```python
from build123d import *

# Parameters (mm, degrees)
F1_DEPTH = 5.08
F3_DEPTH = 751.84


with BuildPart() as f1:
    # F0 (on Front) → F1 (new body)
    with BuildSketch(Plane.XZ):
        Polygon((0, 482.6), (0, 0), (647.7, 0), (647.7, 504.825), align=None)
    extrude(amount=-F1_DEPTH)

    # F2 (on face) → F3 (cut)
    with BuildSketch(Plane.YZ.offset(647.7)):
        Polygon((5.08, 1.116884), (3.951849, 0), (5.08, 0), align=None)
        Polygon((0, 1.122531), (0, 0), (1.122533, 0), align=None)
    extrude(amount=-F3_DEPTH, mode=Mode.SUBTRACT)


solid = f1.part
```
Geometry: final body of the model. Coordinates: model frame, mm. Round coordinates to 2 decimals unless told otherwise and drop trailing zeros. Loops run counter-clockwise (first coordinate to the right, second up) from the corner with the lowest first, then second, coordinate; pieces in that order, holes last.
Item 1: Section B-B, the plane y = 2.95. Output: boundary loops of the cut face in (x, z) (3 decimals), plus the area to 3 significant figures.
Checked values:
outline: (0, 0) - (647.7, 0) - (647.7, 504.825) - (0, 482.6) - close
area: 320,000 mm2
Item 2: Section C-C, the plane x = 230.5. Output: boundary loops of the cut face in (y, z), plus the area to 3 significant figures.
Checked values:
outline: (0, 1.12) - (1.12, 0) - (3.95, 0) - (5.08, 1.12) - (5.08, 490.51) - (0, 490.51) - close
area: 2,490 mm2
Item 3: Line query: L1, parallel to Z at x = 268, y = 3.4; L2, parallel to Z at x = 55.5, y = 3.2. Output: solid intervals per line, ascending.
Checked values:
L1: z = 0 to 491.8
L2: z = 0 to 484.5
Item 4: Section A-A, the plane x = 304. Output: boundary loops of the cut face in (y, z).
Checked values:
outline: (0, 1.12) - (1.12, 0) - (3.95, 0) - (5.08, 1.12) - (5.08, 493.03) - (0, 493.03) - close
Item 5: Contact query for flat-ended pins moving along their axis: P1, Ø1, axis at x = 204, y = 1.5, coming from the -Z side; P2, Ø2, axis at x = 127, y = 1.5, coming from the +Z side; P3, Ø3, axis at x = 509.5, y = 3.5, coming from the +Z side. Output: stop coordinate, or through.
Checked values:
P1: stops at z = 0
P2: stops at z = 486.99
P3: stops at z = 500.13
